from build123d import *

# Parameters (mm, degrees)
SKETCH_1_R      = 3.5
SKETCH_1_R_2    = 2.5
EXTRUDE_1_DEPTH = 1000


with BuildPart() as part:
    # Эскиз1 → Бобышка-Вытянуть1 (new body)
    with BuildSketch(Plane.XY):
        with BuildLine():
            Line((-30, 20.15), (-30, 29.5))
            ThreePointArc((-30, 29.5), (-29.853553391, 29.853553391), (-29.5, 30))
            Line((-29.5, 30), (-20.15, 30))
            Line((-20.15, 30), (-18.15, 30))
            Line((-18.15, 30), (-18.15, 27.5))
            Line((-18.15, 27.5), (-20.15, 27.5))
            Line((-20.15, 27.5), (-20.15, 22.5))
            Line((-20.15, 22.5), (-18.15, 22.5))
            Line((-18.15, 22.5), (-18.15, 20))
            Line((-18.15, 20), (-11.85, 20))
            Line((-11.85, 20), (-11.85, 22.5))
            Line((-11.85, 22.5), (-9.85, 22.5))
            Line((-9.85, 22.5), (-9.85, 27.5))
            Line((-9.85, 27.5), (-11.85, 27.5))
            Line((-11.85, 27.5), (-11.85, 30))
            Line((-11.85, 30), (-9.85, 30))
            Line((-9.85, 30), (0, 30))
            Line((0, 30), (9.85, 30))
            Line((9.85, 30), (11.85, 30))
            Line((11.85, 30), (11.85, 27.5))
            Line((11.85, 27.5), (9.85, 27.5))
            Line((9.85, 27.5), (9.85, 22.5))
            Line((9.85, 22.5), (11.85, 22.5))
            Line((11.85, 22.5), (11.85, 20))
            Line((11.85, 20), (18.15, 20))
            Line((18.15, 20), (18.15, 22.5))
            Line((18.15, 22.5), (20.15, 22.5))
            Line((20.15, 22.5), (20.15, 27.5))
            Line((20.15, 27.5), (18.15, 27.5))
            Line((18.15, 27.5), (18.15, 30))
            Line((18.15, 30), (20.15, 30))
            Line((20.15, 30), (29.5, 30))
            ThreePointArc((29.5, 30), (29.853553391, 29.853553391), (30, 29.5))
            Line((30, 29.5), (30, 20.15))
            Line((30, 20.15), (30, 18.15))
            Line((30, 18.15), (27.5, 18.15))
            Line((27.5, 18.15), (27.5, 20.15))
            Line((27.5, 20.15), (22.5, 20.15))
            Line((22.5, 20.15), (22.5, 18.15))
            Line((22.5, 18.15), (20, 18.15))
            Line((20, 18.15), (20, 11.85))
            Line((20, 11.85), (22.5, 11.85))
            Line((22.5, 11.85), (22.5, 9.85))
            Line((22.5, 9.85), (27.5, 9.85))
            Line((27.5, 9.85), (27.5, 11.85))
            Line((27.5, 11.85), (30, 11.85))
            Line((30, 11.85), (30, 9.85))
            Line((30, 9.85), (30, 0))
            Line((30, 0), (30, -9.85))
            Line((30, -9.85), (30, -11.85))
            Line((30, -11.85), (27.5, -11.85))
            Line((27.5, -11.85), (27.5, -9.85))
            Line((27.5, -9.85), (22.5, -9.85))
            Line((22.5, -9.85), (22.5, -11.85))
            Line((22.5, -11.85), (20, -11.85))
            Line((20, -11.85), (20, -18.15))
            Line((20, -18.15), (22.5, -18.15))
            Line((22.5, -18.15), (22.5, -20.15))
            Line((22.5, -20.15), (27.5, -20.15))
            Line((27.5, -20.15), (27.5, -18.15))
            Line((27.5, -18.15), (30, -18.15))
            Line((30, -18.15), (30, -20.15))
            Line((30, -20.15), (30, -29.5))
            ThreePointArc((30, -29.5), (29.853553391, -29.853553391), (29.5, -30))
            Line((29.5, -30), (20.15, -30))
            Line((20.15, -30), (18.15, -30))
            Line((18.15, -30), (18.15, -27.5))
            Line((18.15, -27.5), (20.15, -27.5))
            Line((20.15, -27.5), (20.15, -22.5))
            Line((20.15, -22.5), (18.15, -22.5))
            Line((18.15, -22.5), (18.15, -20))
            Line((18.15, -20), (11.85, -20))
            Line((11.85, -20), (11.85, -22.5))
            Line((11.85, -22.5), (9.85, -22.5))
            Line((9.85, -22.5), (9.85, -27.5))
            Line((9.85, -27.5), (11.85, -27.5))
            Line((11.85, -27.5), (11.85, -30))
            Line((11.85, -30), (9.85, -30))
            Line((9.85, -30), (0, -30))
            Line((0, -30), (-9.85, -30))
            Line((-9.85, -30), (-11.85, -30))
            Line((-11.85, -30), (-11.85, -27.5))
            Line((-11.85, -27.5), (-9.85, -27.5))
            Line((-9.85, -27.5), (-9.85, -22.5))
            Line((-9.85, -22.5), (-11.85, -22.5))
            Line((-11.85, -22.5), (-11.85, -20))
            Line((-11.85, -20), (-18.15, -20))
            Line((-18.15, -20), (-18.15, -22.5))
            Line((-18.15, -22.5), (-20.15, -22.5))
            Line((-20.15, -22.5), (-20.15, -27.5))
            Line((-20.15, -27.5), (-18.15, -27.5))
            Line((-18.15, -27.5), (-18.15, -30))
            Line((-18.15, -30), (-20.15, -30))
            Line((-20.15, -30), (-29.5, -30))
            ThreePointArc((-29.5, -30), (-29.853553391, -29.853553391), (-30, -29.5))
            Line((-30, -29.5), (-30, -20.15))
            Line((-30, -20.15), (-30, -18.15))
            Line((-30, -18.15), (-27.5, -18.15))
            Line((-27.5, -18.15), (-27.5, -20.15))
            Line((-27.5, -20.15), (-22.5, -20.15))
            Line((-22.5, -20.15), (-22.5, -18.15))
            Line((-22.5, -18.15), (-20, -18.15))
            Line((-20, -18.15), (-20, -11.85))
            Line((-20, -11.85), (-22.5, -11.85))
            Line((-22.5, -11.85), (-22.5, -9.85))
            Line((-22.5, -9.85), (-27.5, -9.85))
            Line((-27.5, -9.85), (-27.5, -11.85))
            Line((-27.5, -11.85), (-30, -11.85))
            Line((-30, -11.85), (-30, -9.85))
            Line((-30, -9.85), (-30, 0))
            Line((-30, 0), (-30, 9.85))
            Line((-30, 9.85), (-30, 11.85))
            Line((-30, 11.85), (-27.5, 11.85))
            Line((-27.5, 11.85), (-27.5, 9.85))
            Line((-27.5, 9.85), (-22.5, 9.85))
            Line((-22.5, 9.85), (-22.5, 11.85))
            Line((-22.5, 11.85), (-20, 11.85))
            Line((-20, 11.85), (-20, 18.15))
            Line((-20, 18.15), (-22.5, 18.15))
            Line((-22.5, 18.15), (-22.5, 20.15))
            Line((-22.5, 20.15), (-27.5, 20.15))
            Line((-27.5, 20.15), (-27.5, 18.15))
            Line((-27.5, 18.15), (-30, 18.15))
            Line((-30, 18.15), (-30, 20.15))
        make_face()
        with Locations((-25, 25)):
            Circle(SKETCH_1_R, mode=Mode.SUBTRACT)
        with Locations((-15, 15)):
            Circle(SKETCH_1_R_2, mode=Mode.SUBTRACT)
        with Locations((25, 25)):
            Circle(SKETCH_1_R, mode=Mode.SUBTRACT)
        with Locations((15, 15)):
            Circle(SKETCH_1_R_2, mode=Mode.SUBTRACT)
        with Locations((25, -25)):
            Circle(SKETCH_1_R, mode=Mode.SUBTRACT)
        with Locations((15, -15)):
            Circle(SKETCH_1_R_2, mode=Mode.SUBTRACT)
        with Locations((-25, -25)):
            Circle(SKETCH_1_R, mode=Mode.SUBTRACT)
        with Locations((-15, -15)):
            Circle(SKETCH_1_R_2, mode=Mode.SUBTRACT)
        with BuildLine():
            Line((0, 27.6), (-5.15, 27.6))
            ThreePointArc((-5.15, 27.6), (-6.988477631, 26.838477631), (-7.75, 25))
            Line((-7.75, 25), (-7.75, 21.1))
            Line((-7.75, 21.1), (-10, 18.1))
            Line((-10, 18.1), (-10, 15))
            ThreePointArc((-10, 15), (-11.464466094, 11.464466094), (-15, 10))
            Line((-15, 10), (-18.1, 10))
            Line((-18.1, 10), (-21.1, 7.75))
            Line((-21.1, 7.75), (-25, 7.75))
            ThreePointArc((-25, 7.75), (-26.838477631, 6.988477631), (-27.6, 5.15))
            Line((-27.6, 5.15), (-27.6, 0))
            Line((-27.6, 0), (-27.6, -5.15))
            ThreePointArc((-27.6, -5.15), (-26.838477631, -6.988477631), (-25, -7.75))
            Line((-25, -7.75), (-21.1, -7.75))
            Line((-21.1, -7.75), (-18.1, -10))
            Line((-18.1, -10), (-15, -10))
            ThreePointArc((-15, -10), (-11.464466094, -11.464466094), (-10, -15))
            Line((-10, -15), (-10, -18.1))
            Line((-10, -18.1), (-7.75, -21.1))
            Line((-7.75, -21.1), (-7.75, -25))
            ThreePointArc((-7.75, -25), (-6.988477631, -26.838477631), (-5.15, -27.6))
            Line((-5.15, -27.6), (0, -27.6))
            Line((0, -27.6), (5.15, -27.6))
            ThreePointArc((5.15, -27.6), (6.988477631, -26.838477631), (7.75, -25))
            Line((7.75, -25), (7.75, -21.1))
            Line((7.75, -21.1), (10, -18.1))
            Line((10, -18.1), (10, -15))
            ThreePointArc((10, -15), (11.464466094, -11.464466094), (15, -10))
            Line((15, -10), (18.1, -10))
            Line((18.1, -10), (21.1, -7.75))
            Line((21.1, -7.75), (25, -7.75))
            ThreePointArc((25, -7.75), (26.838477631, -6.988477631), (27.6, -5.15))
            Line((27.6, -5.15), (27.6, 0))
            Line((27.6, 0), (27.6, 5.15))
            ThreePointArc((27.6, 5.15), (26.838477631, 6.988477631), (25, 7.75))
            Line((25, 7.75), (21.1, 7.75))
            Line((21.1, 7.75), (18.1, 10))
            Line((18.1, 10), (15, 10))
            ThreePointArc((15, 10), (11.464466094, 11.464466094), (10, 15))
            Line((10, 15), (10, 18.1))
            Line((10, 18.1), (7.75, 21.1))
            Line((7.75, 21.1), (7.75, 25))
            ThreePointArc((7.75, 25), (6.988477631, 26.838477631), (5.15, 27.6))
            Line((5.15, 27.6), (0, 27.6))
        make_face(mode=Mode.SUBTRACT)
    extrude(amount=EXTRUDE_1_DEPTH)


solid = part.part
The listing builds one solid part. Answer for the finished solid, in the listing's coordinates (mm). Give positions to 0.01 mm unless a question says otherwise; leave off trailing zeros.
1) Find the intervals of material crossed by L1, parallel to Y at x = -25, z = 207; L2, parallel to Y at x = -15, z = 260, in increasing order.
2) Section A-A (z = 89.5) is taken. Count the separate pieces of the cut face and the enclosed holes in it, and give its area (3 significant figures).
3) Given P1, Ø6, axis at x = -5, y = -16.5, coming from the -Z side; P2, Ø0.9, axis at y = -17, z = 315, coming from the -X side; P3, Ø1.5, axis at y = -14.5, z = 659, coming from the +X side, each flat-ended and moving along its own axis, determine where each tip first touches the part or whether it passes through.
Response:
1. L1: y = -30 to -28.5, -21.5 to -20.15, -9.85 to -7.75, 7.75 to 9.85, 20.15 to 21.5, 28.5 to 30
1. L2: y = -20 to -17.5, -12.5 to -10, 10 to 12.5, 17.5 to 20
2. separate pieces: 1
2. enclosed holes: 9
2. area: 1,030 mm2
3. P1: passes through
3. P2: stops at x = -20
3. P3: stops at x = 20
